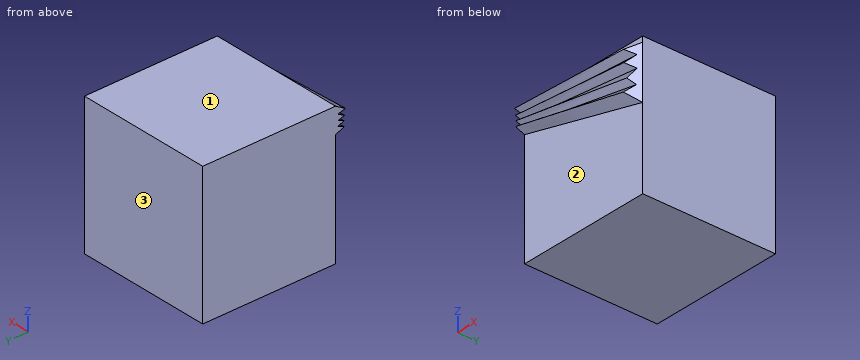
```python
from build123d import *

# Parameters (mm, degrees)
F0_W     = 81.678458
F0_H     = 80.120139
F1_DEPTH = 83.81969
F6_DEPTH = 83.82069


with BuildPart() as f1:
    # F0 (on Top) → F1 (new body)
    with BuildSketch(Plane.XY):
        with Locations((40.839229, 40.060069)):
            Rectangle(F0_W, F0_H)
    extrude(amount=F1_DEPTH)

    # F2 (on face) → F4 section 0
    with BuildSketch(Plane.YZ.offset(81.678458)):
        Polygon((0, 48.545107), (0, 80.539919), (-6.469702, 76.612413), (-1.871645, 73.930211), (-6.37391, 69.332153), (-1.871645, 66.554159), (-5.404703, 60.828167), (-2.06323, 57.741221), (-6.575088, 52.857349), align=None)
    # F3 (on face) → F4 section 1
    with BuildSketch(Plane(origin=(0, 0, 0), x_dir=(0, -1, 0), z_dir=(-1, 0, 0))):
        Polygon((6.032056, 80.237612), (0, 83.81969), (0, 68.663813), (5.409211, 70.837572), (1.381365, 72.499856), (5.153475, 74.034274), (1.381365, 75.568691), (5.53708, 76.7195), (1.381365, 79.021126), align=None)
    loft()

    # F5 (on face) → F6 (cut, through all)
    with BuildSketch(Plane.XY.offset(83.81969)):
        Polygon((83.874113, -8.362563), (81.678458, 0), (73.979422, -8.362563), align=None)
    extrude(amount=-F6_DEPTH, mode=Mode.SUBTRACT)


solid = f1.part
```
The model under review builds one solid part; all positions refer to its coordinate system, in mm. Face numbers are marked on the shaded views. Round coordinates to 2 decimals unless told otherwise and drop trailing zeros. Order: outer loops, then holes, each group sorted by start corner. A loop starts at its lowest first (then second) coordinate and runs counter-clockwise, first axis right, second up. Notation, with made-up numbers: M -19,4 L 29,4 A19 ccw 29,27 Z; hole C 88,21 d4. An arc over 180 degrees is marked long. Use a Markdown table: item, result.
1) Draft analysis for pull direction Y (two halves, no side actions). For the marked faces 1, 2 and 3, state which applies: released by +Y, released by -Y, zero draft, split by the parting line, or undercut.
Report:
| item | result |
|---|---|
| face 1 | zero draft |
| face 2 | released by -Y |
| face 3 | released by +Y |
2) Insertion check: pin 1 (1.5 mm diameter, centred on x = 19.5, z = 19, fed in from -Y); pin 2 (1.6 mm diameter, centred on x = 28.5, z = 82.5, fed in from -Y); pin 3 (8 mm diameter, centred on x = 20, y = 20, fed in from -Z). Each pin has a flat end and moves straight along its axis. Give the tip position at first contact, or say it passes through.
Report:
| item | result |
|---|---|
| pin 1 | y = 0 |
| pin 2 | y = -1.63 |
| pin 3 | z = 0 |
3) Consider section A-A (z = 15.5). Write out the cut boundary in (x, y), then the cut area to 3 significant figures.
Report:
| item | result |
|---|---|
| outline | M 0,0 L 81.68,0 L 81.68,80.12 L 0,80.12 Z |
| area | 6,540 mm^2 |
4) Wall thickness on line 1 along Y through (x, z) = (66.5, 32.5); line 2 along Y through (x, z) = (59.5, 56): over which ranges is each line inside the solid? List them lowest first. Write a range as [from, to].
Report:
| item | result |
|---|---|
| line 1 | [0, 80.12] |
| line 2 | [-3.34, 80.12] |
